from build123d import *

# Parameters (mm, degrees)
BOSS_EXTRUDE1_DEPTH      = 16
SKETCH2_W                = 21
SKETCH2_H                = 8
CUT_EXTRUDE1_DEPTH       = 44.0464865
SKETCH3_R                = 9.5
CUT_EXTRUDE2_DEPTH       = 36.0142828
FILLET1_R                = 16
F_3_0_3_DIAMETER_HOLE1_D = 3
SKETCH6_W                = 9
SKETCH6_H                = 8
CUT_EXTRUDE3_DEPTH       = 36.0142828
FILLET2_R                = 3


with BuildPart() as part:
    # Sketch1 → Boss-Extrude1 (new, symmetric)
    with BuildSketch(Plane(origin=(0, 0, 0), x_dir=(1, 0, 0), z_dir=(0, 1, 0))):
        Polygon((-17, 0), (17, 0), (17, 4), (-23, 4), (-23, -21), (-17, -21), align=None)
    extrude(amount=BOSS_EXTRUDE1_DEPTH, both=True)

    # Sketch2 → Cut-Extrude1 (cut, through all)
    with BuildSketch(Plane(origin=(-17, 0, 0), x_dir=(0, 0, -1), z_dir=(1, 0, 0))):
        with Locations((-10.5, 12)):
            Rectangle(SKETCH2_W, SKETCH2_H)
        with Locations((-10.5, -12)):
            Rectangle(SKETCH2_W, SKETCH2_H)
    extrude(amount=-CUT_EXTRUDE1_DEPTH, mode=Mode.SUBTRACT)

    # Sketch3 → Cut-Extrude2 (cut, through all)
    with BuildSketch(Plane.XY):
        Circle(SKETCH3_R)
    extrude(amount=-CUT_EXTRUDE2_DEPTH, mode=Mode.SUBTRACT)

    # Fillet1
    fillet1_edges = [part.edges().sort_by_distance(p)[0] for p in [
        (17, -16, -2),
        (17, 16, -2),
    ]]
    fillet(fillet1_edges, radius=FILLET1_R - 0.0001)  # a hair under: the kernel refuses the full size

    # Ø3.0 (3) Diameter Hole1 (through all)
    with Locations(Plane(origin=(0, 0, -4), x_dir=(-1, 0, 0), z_dir=(0, 0, -1))):
        with Locations((0, 13), (13, 0), (0, -13), (-13, 0)):
            Hole(F_3_0_3_DIAMETER_HOLE1_D / 2)

    # Sketch6 → Cut-Extrude3 (cut, through all)
    with BuildSketch(Plane.XY):
        with Locations((-18.5, -12)):
            Rectangle(SKETCH6_W, SKETCH6_H)
    extrude(amount=-CUT_EXTRUDE3_DEPTH, mode=Mode.SUBTRACT)

    # Fillet2
    fillet2_edges = [part.edges().sort_by_distance(p)[0] for p in [
        (-14, -16, -2),
        (-14, -8, -2),
    ]]
    fillet(fillet2_edges, radius=FILLET2_R)


solid = part.part
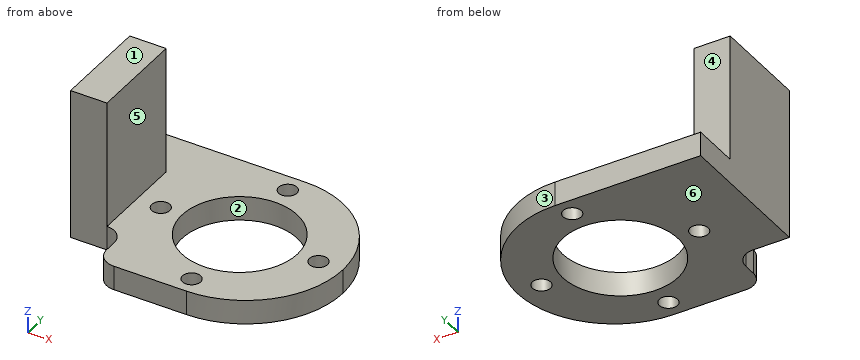
For this review, take the finished solid that the model builds, in its own axes (mm). Face numbers are marked on the shaded views. A direction names the side the tool comes from. Coordinates: 2 decimals unless noted, no trailing zeros. Loops run counter-clockwise (first coordinate to the right, second up) from the corner with the lowest first, then second, coordinate; pieces in that order, holes last. Notation, with made-up numbers: (59, 48) -> (63, 48) arc R27 cw to (63, 81) -> close; hole circle Ø6 at (-28, -35.75). An arc over 180 degrees is marked (long way). Write each question's results on one line, items separated by ' | '.
Q1. To check wall thickness, follow line 1 along Y through (x, z) = (0, -1.7); line 2 along Z through (x, y) = (-3, 14.5); line 3 along X through (y, z) = (-2.5, -2.5). State the ranges of each line that lie inside material, in increasing order. Write a range as [from, to].
Taken from the geometry:
line 1: [-16, -14.5], [-11.5, -9.5], [9.5, 11.5], [14.5, 16] | line 2: [-4, 0] | line 3: [-23, -9.17], [9.17, 16.8]
Q2. Mouldability with a two-part tool opening along Y and no side actions: class the marked faces 1, 2 and 3 as +Y half, -Y half, draft (parallel to the pull), parting line (faces both ways), or undercut.
Taken from the geometry:
face 1: draft | face 2: undercut | face 3: +Y half
Q3. Add section D-D, the plane x = -19. State the section outline as (y, z) points.
Taken from the geometry:
outline: (-8, -4) -> (16, -4) -> (16, 0) -> (8, 0) -> (8, 21) -> (-8, 21) -> close
Q4. Machinability: for the marked faces 4, 5 and 6, which of the approach directions +Z, -Z, +X, -X, +Y, -Y give a long, thin tool a straight path to every point of the face, cutting with its end or side? Answer none if there is none.
Taken from the geometry:
face 4: +Z, +X, -X, +Y | face 5: +Z, +X, +Y, -Y | face 6: -Z, +X, -X, +Y, -Y
Q5. Add section A-A, the plane x = 0. State the section outline as (y, z) points, then the cut area to 3 significant figures.
Taken from the geometry:
outline: (-16, -4) -> (-14.5, -4) -> (-14.5, 0) -> (-16, 0) -> close; (-11.5, -4) -> (-9.5, -4) -> (-9.5, 0) -> (-11.5, 0) -> close; (9.5, -4) -> (11.5, -4) -> (11.5, 0) -> (9.5, 0) -> close; (14.5, -4) -> (16, -4) -> (16, 0) -> (14.5, 0) -> close | area: 28.0 mm²
Q6. Add section B-B, the plane y = 7. State the section outline as (x, z) points.
Taken from the geometry:
outline: (-23, -4) -> (-6.42, -4) -> (-6.42, 0) -> (-17, 0) -> (-17, 21) -> (-23, 21) -> close; (6.42, -4) -> (15.39, -4) -> (15.39, 0) -> (6.42, 0) -> close
Q7. For pin 1 Ø5 at (x, y) = (0, 13) entering from +Z; pin 2 Ø0.6 at (y, z) = (-11.5, -2) entering from -X; pin 3 Ø8 at (x, z) = (9.5, 6.5) entering from +Y; pin 4 Ø6.5 at (x, z) = (-21, 11) entering from +Y, all flat-tipped, find the tip position at first contact; note any pin that passes through.
Taken from the geometry:
pin 1: z = 0 | pin 2: x = -14 | pin 3: through | pin 4: y = 8
Q8. Add section C-C, the plane x = -6. State the section outline as (y, z) points.
Taken from the geometry:
outline: (-16, -4) -> (-7.37, -4) -> (-7.37, 0) -> (-16, 0) -> close; (7.37, -4) -> (16, -4) -> (16, 0) -> (7.37, 0) -> close
